```python
from build123d import *

# Parameters (mm, degrees)
F2_SIZE = 5.08
F3_R    = 15.24


with BuildPart() as f1:
    # F0 (on Top) → F1 (revolve)
    with BuildSketch(Plane.XY):
        Polygon((-46.351972, 43.938525), (0, 0), (0, 50.97072), align=None)
        Polygon((0, 50.97072), (0, 0), (119.629055, 0), (119.629055, 50.97072), (95.021219, 74.297279), (22.111996, 74.297279), align=None)
    revolve(axis=Axis((59.814528, 0, 0), (-1, 0, 0)))

    # F2
    f2_edges = [f1.edges().sort_by_distance(p)[0] for p in [
        (95.021219, -74.297279, 0),
    ]]
    chamfer(f2_edges, length=F2_SIZE)

    # F3
    f3_edges = [f1.edges().sort_by_distance(p)[0] for p in [
        (119.629055, -50.97072, 0),
    ]]
    fillet(f3_edges, radius=F3_R)


solid = f1.part
```
The model under review builds one solid part; all positions refer to its coordinate system, in mm. Round coordinates to 2 decimals unless told otherwise and drop trailing zeros. Order: outer loops, then holes, each group sorted by start corner. A loop starts at its lowest first (then second) coordinate and runs counter-clockwise, first axis right, second up. Notation, with made-up numbers: (-28, 47.5) -> (-19, 47.5) arc R15 ccw to (-19, 58.5) -> close; hole circle Ø11 at (74, 62.25). An arc over 180 degrees is marked (long way). One line per item, written item: value. Start each with the question number.
Q1. Clearance check with flat-ended pins moving along their axes: pin 1 Ø5 at (x, y) = (61, 20.5) entering from +Z; pin 2 Ø2 at (x, z) = (-9, 26.5) entering from +Y; pin 3 Ø1 at (x, z) = (76.5, 21.5) entering from +Y. State where each tip first meets the part, or that it passes through.
Q2. Take a section at B-B (x = 3). Write out the cut boundary in (y, z), and give its area (3 significant figures).
Q3. Mouldability with a two-part tool opening along Y and no side actions: class faces 1 (the face through (-12.55, 11.35, -3.57)), 2 (the face through (113.86, -12.23, 55.1)), 3 (the face through (119.629, 1, -1)) as released by +Y, released by -Y, zero draft, split by the parting line, or undercut.
Q4. Take a section at A-A (x = 32). Write out the cut boundary in (y, z), and give its area (3 significant figures).
Q5. Wall thickness on line 1 (Z direction, x = -21, y = -13); line 2 (Z direction, x = -38.5, y = -23.5); line 3 (Y direction, x = 2, z = 20): over which ranges is each line inside the solid? List them lowest first.
Reported:
1. pin 1: stops at z = 72.08
1. pin 2: stops at y = 42.57
1. pin 3: stops at y = 71.27
2. outline: circle Ø108.27 at (0, 0)
2. area: 9,210 mm2
3. face 1: undercut
3. face 2: split by the parting line
3. face 3: zero draft
4. outline: circle Ø148.59 at (0, 0)
4. area: 17,300 mm2
5. line 1: z = -45.98 to -15.08, 15.08 to 45.98
5. line 2: z = -38.53 to -27.92, 27.92 to 38.53
5. line 3: y = -49.17 to 49.17
